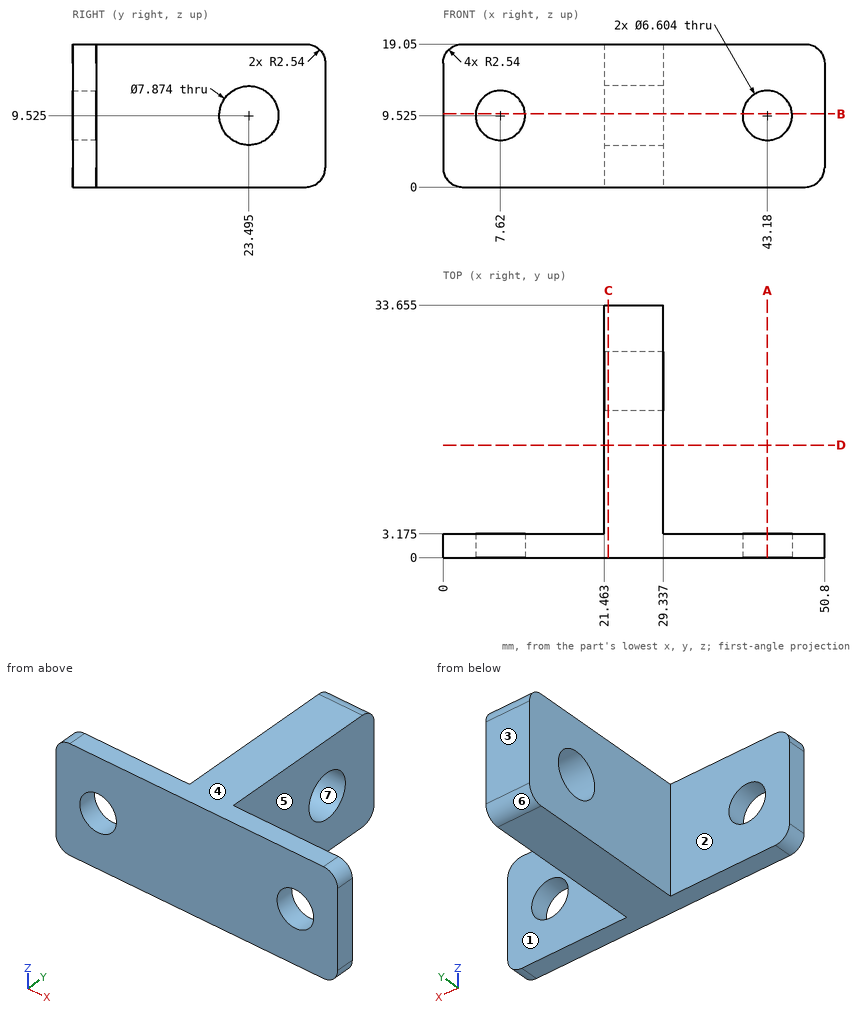
For this review, use the dimensioned drawing (mm, ordinates from the lowest corner) and the shaded views. A direction names the side the tool comes from. Round coordinates to 2 decimals unless told otherwise and drop trailing zeros. Order: outer loops, then holes, each group sorted by start corner. A loop starts at its lowest first (then second) coordinate and runs counter-clockwise, first axis right, second up.
1) Consider section C-C (x = 22). State the section outline as (y, z) points (3 decimals), plus the area to 3 significant figures.
The answers:
outline: (0, 0) - (31.115, 0) arc R2.54 ccw to (33.655, 2.54) - (33.655, 16.51) arc R2.54 ccw to (31.115, 19.05) - (0, 19.05) - close; hole circle Ø7.874 at (23.495, 9.525)
area: 590 mm2
2) Consider section D-D (y = 15). State the section outline as (x, z) points, plus the area to 3 significant figures.
The answers:
outline: (21.46, 0) - (29.34, 0) - (29.34, 19.05) - (21.46, 19.05) - close
area: 150 mm2
3) Consider section A-A (x = 43.18). State the section outline as (y, z) points (3 decimals), plus the area to 3 significant figures.
The answers:
outline: (0, 0) - (3.175, 0) - (3.175, 6.223) - (0, 6.223) - close; (0, 12.827) - (3.175, 12.827) - (3.175, 19.05) - (0, 19.05) - close
area: 39.5 mm2
4) Draft analysis for pull direction Z (two halves, no side actions). For the marked faces 4, 5, 6 and 7, state which applies: released by +Z, released by -Z, zero draft, split by the parting line, or undercut.
The answers:
face 4: released by +Z
face 5: zero draft
face 6: released by -Z
face 7: undercut
5) Machinability: for the marked faces 1, 2 and 3, which of the approach directions +Z, -Z, +X, -X, +Y, -Y give a long, thin tool a straight path to every point of the face, cutting with its end or side? Answer none if there is none.
The answers:
face 1: +Z, -Z, +X, +Y
face 2: +Z, -Z, -X, +Y
face 3: +Z, -Z, +X, -X, +Y
6) Clearance check with flat-ended pins moving along their axes: pin 1 Ø10 at (y, z) = (23.495, 9.525) entering from -X; pin 2 Ø9.5 at (x, z) = (13, 11) entering from +Y (3 decimals); pin 3 Ø10 at (y, z) = (10, 5) entering from +X. State where each tip first meets the part, or that it passes through.
The answers:
pin 1: stops at x = 21.46
pin 2: stops at y = 3.175
pin 3: stops at x = 29.34
7) Consider section B-B (z = 9.75). State the section outline as (x, y) points (3 decimals), plus the area to 3 significant figures.
The answers:
outline: (0, 0) - (4.326, 0) - (4.326, 3.175) - (0, 3.175) - close; (10.914, 0) - (39.886, 0) - (39.886, 3.175) - (29.337, 3.175) - (29.337, 19.564) - (21.463, 19.564) - (21.463, 3.175) - (10.914, 3.175) - close; (21.463, 27.426) - (29.337, 27.426) - (29.337, 33.655) - (21.463, 33.655) - close; (46.474, 0) - (50.8, 0) - (50.8, 3.175) - (46.474, 3.175) - close
area: 298 mm2
8) For L1, parallel to Z at x = 43, y = 1; L2, parallel to Y at x = 39, z = 6.25 (3 decimals); L3, parallel to X at y = 5.5, z = 3, list the stretches that pass through material, from the lowest coordinate up.
The answers:
L1: z = 0 to 6.23, 12.82 to 19.05
L2: y = 0 to 3.175
L3: x = 21.46 to 29.34
